```python
from build123d import *

# Parameters (mm, degrees)
SKETCH1_W                = 80
SKETCH1_H                = 80
BOSS_EXTRUDE1_DEPTH      = 12
CHAMFER1_SIZE            = 3
CUT_EXTRUDE1_DEPTH       = 6
MIRROR2_COPY_1_DEPTH     = 6
HOLE3_D                  = 5
HOLE3_CBORE_D            = 9
HOLE3_CBORE_DEPTH        = 4
SKETCH9_R                = 15
BOSS_EXTRUDE2_DEPTH      = 6
CUT_EXTRUDE2_DEPTH       = 60.363288319
CIRPATTERN1_COUNT        = 4
BOSS_EXTRUDE3_START      = 5
BOSS_EXTRUDE3_DEPTH      = 0.75
CIRPATTERN2_COUNT        = 4
CIRPATTERN2_START        = 5
CIRPATTERN2_COPY_1_DEPTH = 0.75
CIRPATTERN2_COPY_2_DEPTH = 0.75
CIRPATTERN2_COPY_3_DEPTH = 0.75
HOLE4_D                  = 20


with BuildPart() as part:
    # Sketch1 → Boss-Extrude1 (new body)
    with BuildSketch(Plane(origin=(0, 0, 0), x_dir=(1, 0, 0), z_dir=(0, 1, 0))):
        Rectangle(SKETCH1_W, SKETCH1_H)
    extrude(amount=BOSS_EXTRUDE1_DEPTH)

    # Chamfer1
    chamfer1_edges = [part.edges().sort_by_distance(p)[0] for p in [
        (40, 6, 40),
        (-40, 6, 40),
        (-40, 6, -40),
        (40, 6, -40),
    ]]
    chamfer(chamfer1_edges, length=CHAMFER1_SIZE)

    # Sketch2 → Cut-Extrude1 (cut)
    with BuildSketch(Plane(origin=(0, 12, 0), x_dir=(1, 0, 0), z_dir=(0, 1, 0))):
        with BuildLine():
            Line((-40, -24), (-32, -24))
            ThreePointArc((-32, -24), (-26.343145751, -26.343145751), (-24, -32))
            Line((-24, -32), (-24, -40))
            Line((-24, -40), (-37, -40))
            Line((-37, -40), (-40, -37))
            Line((-40, -37), (-40, -24))
        make_face()
    cut_extrude1 = extrude(amount=-CUT_EXTRUDE1_DEPTH, mode=Mode.SUBTRACT)

    # Mirror1: Cut-Extrude1 across plane
    add(cut_extrude1.mirror(Plane(origin=(0, 0, 0), x_dir=(0, 0, 1), z_dir=(1, 0, 0))), mode=Mode.SUBTRACT)

    # Mirror2: Cut-Extrude1 across plane
    add(cut_extrude1.mirror(Plane.XY), mode=Mode.SUBTRACT)

    # Mirror2 copy 1 sketch → Mirror2 copy 1 (cut)
    with BuildSketch(Plane(origin=(0, 12, 0), x_dir=(-1, 0, 0), z_dir=(0, 1, 0))):
        with BuildLine():
            Line((-40, -24), (-32, -24))
            ThreePointArc((-32, -24), (-26.343145751, -26.343145751), (-24, -32))
            Line((-24, -32), (-24, -40))
            Line((-24, -40), (-37, -40))
            Line((-37, -40), (-40, -37))
            Line((-40, -37), (-40, -24))
        make_face()
    extrude(amount=-MIRROR2_COPY_1_DEPTH, mode=Mode.SUBTRACT)

    # Hole3 (through all)
    with Locations(Plane(origin=(0, 6, 0), x_dir=(1, 0, 0), z_dir=(0, 1, 0))):
        with Locations((-32, -32), (32, -32), (32, 32), (-32, 32)):
            CounterBoreHole(HOLE3_D / 2, HOLE3_CBORE_D / 2, HOLE3_CBORE_DEPTH)

    # Sketch9 → Boss-Extrude2 (add)
    with BuildSketch(Plane(origin=(0, 12, 0), x_dir=(1, 0, 0), z_dir=(0, 1, 0))):
        with Locations(Location((0, 0, 0), (0, 0, 270))):
            Circle(SKETCH9_R)
    extrude(amount=BOSS_EXTRUDE2_DEPTH)

    # Sketch10 → Cut-Extrude2 (cut, through all)
    with BuildSketch(Plane(origin=(0, 18, 0), x_dir=(1, 0, 0), z_dir=(0, 1, 0))):
        with BuildLine():
            Line((-21, 37), (-21, 32))
            Line((-21, 32), (-5.978240283, 16.978240283))
            ThreePointArc((-5.978240283, 16.978240283), (0, 18), (5.978240283, 16.978240283))
            Line((5.978240283, 16.978240283), (21, 32))
            Line((21, 32), (21, 37))
            Line((21, 37), (-21, 37))
        make_face()
    cut_extrude2 = extrude(amount=-CUT_EXTRUDE2_DEPTH, mode=Mode.SUBTRACT)

    # CirPattern1: Cut-Extrude2 ×4 about axis
    cirpattern1_axis = Axis((0, 0, 0), (0, 1, 0))
    for i in range(1, CIRPATTERN1_COUNT):
        add(cut_extrude2.rotate(cirpattern1_axis, i * 360 / CIRPATTERN1_COUNT), mode=Mode.SUBTRACT)

    # Sketch12 → Boss-Extrude3 (add, symmetric)
    with BuildSketch(Plane(origin=(0, 0, 0), x_dir=(0.7071067811865491, 0, -0.707106781186546), z_dir=(0.707106781186546, 0, 0.7071067811865491)).offset(BOSS_EXTRUDE3_START)):
        Polygon((12, 12), (32, 12), (15, 16), (12, 16), align=None)
    boss_extrude3 = extrude(amount=BOSS_EXTRUDE3_DEPTH, both=True)

    # Mirror4: Boss-Extrude3 across plane
    add(boss_extrude3.mirror(Plane(origin=(0, 0, 0), x_dir=(-0.7071067811865492, 0, 0.7071067811865459), z_dir=(0.707106781186546, 0, 0.7071067811865491))))

    # CirPattern2: Boss-Extrude3 ×4 about axis
    cirpattern2_axis = Axis((0, 0, 0), (0, 1, 0))
    for i in range(1, CIRPATTERN2_COUNT):
        add(boss_extrude3.rotate(cirpattern2_axis, i * 360 / CIRPATTERN2_COUNT))

    # CirPattern2 copy 1 sketch → CirPattern2 copy 1 (add, symmetric)
    with BuildSketch(Plane(origin=(0, 0, 0), x_dir=(-0.707106781186546, 0, -0.7071067811865491), z_dir=(-0.7071067811865493, 0, 0.7071067811865462)).offset(CIRPATTERN2_START)):
        Polygon((12, -12), (32, -12), (15, -16), (12, -16), align=None)
    extrude(amount=CIRPATTERN2_COPY_1_DEPTH, both=True)

    # CirPattern2 copy 2 sketch → CirPattern2 copy 2 (add, symmetric)
    with BuildSketch(Plane(origin=(0, 0, 0), x_dir=(-0.7071067811865492, 0, 0.707106781186546), z_dir=(0.7071067811865461, 0, 0.7071067811865493)).offset(CIRPATTERN2_START)):
        Polygon((12, -12), (32, -12), (15, -16), (12, -16), align=None)
    extrude(amount=CIRPATTERN2_COPY_2_DEPTH, both=True)

    # CirPattern2 copy 3 sketch → CirPattern2 copy 3 (add, symmetric)
    with BuildSketch(Plane(origin=(0, 0, 0), x_dir=(0.707106781186546, 0, 0.7071067811865492), z_dir=(0.7071067811865493, 0, -0.7071067811865461)).offset(CIRPATTERN2_START)):
        Polygon((12, -12), (32, -12), (15, -16), (12, -16), align=None)
    extrude(amount=CIRPATTERN2_COPY_3_DEPTH, both=True)

    # Hole4 (through all)
    with Locations(Plane(origin=(0, 18, 0), x_dir=(1, 0, 0), z_dir=(0, 1, 0))):
        with Locations((0, 0)):
            Hole(HOLE4_D / 2)


solid = part.part
```
Read the model definition and answer for the solid it produces. Units are mm, in the model's axes. A direction names the side the tool comes from. Coordinates: 2 decimals unless noted, no trailing zeros. Loops run counter-clockwise (first coordinate to the right, second up) from the corner with the lowest first, then second, coordinate; pieces in that order, holes last. Notation, with made-up numbers: (-1, -7) -> (23, -7) arc R19 ccw to (23, 18) -> close; hole circle Ø4 at (83.25, -39). An arc over 180 degrees is marked (long way). Return JSON: item names as keys, results as strings.
Item 1: Find section A-A (x = -30.5). Determine the outline of the cut face in (y, z), plus the area to 3 significant figures.
Answers:
{"outline": "(0, -40) -> (6, -40) -> (6, -36.24) -> (2, -36.24) -> (2, -34) -> (0, -34) -> close; (0, -30) -> (2, -30) -> (2, -27.76) -> (6, -27.76) -> (6, -24.14) -> (12, -24.14) -> (12, -19.5) -> (0, -19.5) -> close; (0, 19.5) -> (12, 19.5) -> (12, 24.14) -> (6, 24.14) -> (6, 27.76) -> (2, 27.76) -> (2, 30) -> (0, 30) -> close; (0, 34) -> (2, 34) -> (2, 36.24) -> (6, 36.24) -> (6, 40) -> (0, 40) -> close", "area": "218 mm2"}
Item 2: Find section B-B (z = 0). Determine the outline of the cut face in (x, y), plus the area to 3 significant figures.
Answers:
{"outline": "(-40, 0) -> (-37, 0) -> (-37, 12) -> (-40, 12) -> close; (-18, 0) -> (-10, 0) -> (-10, 18) -> (-15, 18) -> (-15, 12) -> (-18, 12) -> close; (10, 0) -> (18, 0) -> (18, 12) -> (15, 12) -> (15, 18) -> (10, 18) -> close; (37, 0) -> (40, 0) -> (40, 12) -> (37, 12) -> close", "area": "324 mm2"}
Item 3: For a pull along X with two mould halves and no side action, classify faces 1 (the cylindrical face through (26.406, 9.042, -26.281)), 2 (the flat face through (-36, 9, 24)), 3 (the flat face through (-18.76, 13.58, 10.63)), 4 (the flat face through (14, 6, 25)) as +X half, -X half, draft (parallel to the pull), parting line (faces both ways), or undercut.
Answers:
{"face 1": "+X half", "face 2": "draft", "face 3": "-X half", "face 4": "undercut"}
Item 4: Find section D-D (y = 10.5). Count the separate pieces of the cut face and the enclosed holes in it, plus the area to 3 significant figures.
Answers:
{"separate pieces": "1", "enclosed holes": "5", "area": "2,690 mm2"}
Item 5: Find the intervals of material crossed by probe 1 along X at (y, z) = (4.3, -32); probe 2 along X at (y, z) = (0.9, 32); probe 3 along Z at (x, y) = (20.5, 6.25), in increasing order.
Answers:
{"probe 1": "x = -40 to -36.5, -27.5 to -21, 21 to 27.5, 36.5 to 40", "probe 2": "x = -40 to -34.5, -29.5 to -21, 21 to 29.5, 34.5 to 40", "probe 3": "z = -40 to -37, -31.5 to -9.5, 9.5 to 31.5, 37 to 40"}
Item 6: For faces 5 (the flat face through (39, 3, 38)), 6 (the flat face through (36, 9, 24)), 7 (the cylindrical face through (0, 6, -18)), 8 (the cylindrical face through (-27.84, 4.03, 33.72)), 9 (the flat face through (-35.4, 6, 35.4)), determine the directions among +Z, -Z, +X, -X, +Y, -Y from which every point of the face is accessible in a straight line to the end or side of a thin tool.
Answers:
{"face 5": "+Z, +X, +Y, -Y", "face 6": "+Z, +X, +Y", "face 7": "+Y, -Y", "face 8": "+Y", "face 9": "+Z, -X, +Y"}
Item 7: Flat-ended cylindrical pins translate along their axes: P1, Ø6.5, axis at y = 10, z = -34.5, coming from the +X side; P2, Ø13, axis at x = -35, z = 33, coming from the +Y side; P3, Ø1.2, axis at x = -7, z = -14, coming from the +Y side; P4, Ø12, axis at x = 19, z = 17, coming from the -Y side. Find the tip coordinate at first contact, or state that the pin passes through.
Answers:
{"P1": "stops at x = 24.04", "P2": "stops at y = 6", "P3": "stops at y = 16", "P4": "stops at y = 0"}
Item 8: Find section C-C (z = 16). Determine the outline of the cut face in (x, y), plus the area to 3 significant figures.
Answers:
{"outline": "(-40, 0) -> (-37, 0) -> (-37, 12) -> (-40, 12) -> close; (-27, 0) -> (27, 0) -> (27, 12) -> (24.13, 12) -> (24.13, 12.85) -> (22.01, 13.21) -> (22.01, 12) -> (9.99, 12) -> (9.99, 15.21) -> (7.87, 15.56) -> (7.87, 12) -> (-7.87, 12) -> (-7.87, 15.56) -> (-9.99, 15.21) -> (-9.99, 12) -> (-22.01, 12) -> (-22.01, 13.21) -> (-24.13, 12.85) -> (-24.13, 12) -> (-27, 12) -> close; (37, 0) -> (40, 0) -> (40, 12) -> (37, 12) -> close", "area": "739 mm2"}
